Design review of the part built by this model. Coordinates are the model's own, in mm. A direction names the side the tool comes from. Give positions to 0.01 mm unless a question says otherwise; leave off trailing zeros. Loops run counter-clockwise (first coordinate to the right, second up) from the corner with the lowest first, then second, coordinate; pieces in that order, holes last. Notation, with made-up numbers: (-25.75, 79) - (1.25, 79) arc R14 ccw to (1.25, 84) - close; hole circle Ø11 at (64, 24). An arc over 180 degrees is marked (long way). Write each question's results on one line, items separated by ' | '.
from build123d import *

# Parameters (mm, degrees)
SKETCH_1_W          = 35.5
SKETCH_1_H          = 11
SKETCH_1_W_2        = 18.5
SKETCH_1_H_2        = 1.7
CUT_EXTRUDE_1_REACH = 79.86
SKETCH_2_R          = 1.5
CUT_EXTRUDE_START   = -4.5
CUT_EXTRUDE_3_DEPTH = 4.5
SKETCH_4_R          = 2
SKETCH_4_R_2        = 1.5
CUT_EXTRUDE_4_DEPTH = 5


with BuildPart() as part:
    # 草图1 → 旋转1 (revolve)
    with BuildSketch(Plane(origin=(0, 0, 0), x_dir=(1, 0, 0), z_dir=(0, 1, 0))):
        Polygon((0, 24.5), (0, 0), (35.5, 0), (49, 0), (49, 24.5), (24, 24.5), align=None)
        with Locations((17.75, -5.5)):
            Rectangle(SKETCH_1_W, SKETCH_1_H)
        Polygon((0, 25.8), (0, 24.5), (24, 24.5), (24, 25.8), (18.5, 25.8), align=None)
        with Locations((9.25, 26.65)):
            Rectangle(SKETCH_1_W_2, SKETCH_1_H_2)
    revolve(axis=Axis((0, 0, 11), (0, 0, -1)))

    # 草图2 → 切除-拉伸1 (cut, up to next)
    with BuildSketch(Plane(origin=(0, 0, -24.5), x_dir=(-1, 0, 0), z_dir=(0, 0, -1)), mode=Mode.PRIVATE) as cut_extrude_1_sk1:
        with Locations((16.264045876, 39.264880132)):
            Circle(SKETCH_2_R)
    cut_extrude_1_tool1 = extrude(cut_extrude_1_sk1.sketch, amount=-CUT_EXTRUDE_1_REACH, mode=Mode.PRIVATE) & part.part
    # 草图2 → 切除-拉伸1 (cut, up to next)
    with BuildSketch(Plane(origin=(0, 0, -24.5), x_dir=(-1, 0, 0), z_dir=(0, 0, -1)), mode=Mode.PRIVATE) as cut_extrude_1_sk2:
        with Locations((-16.264045876, 39.264880132)):
            Circle(SKETCH_2_R)
    cut_extrude_1_tool2 = extrude(cut_extrude_1_sk2.sketch, amount=-CUT_EXTRUDE_1_REACH, mode=Mode.PRIVATE) & part.part
    # 草图2 → 切除-拉伸1 (cut, up to next)
    with BuildSketch(Plane(origin=(0, 0, -24.5), x_dir=(-1, 0, 0), z_dir=(0, 0, -1)), mode=Mode.PRIVATE) as cut_extrude_1_sk3:
        with Locations((-39.264880132, 16.264045876)):
            Circle(SKETCH_2_R)
    cut_extrude_1_tool3 = extrude(cut_extrude_1_sk3.sketch, amount=-CUT_EXTRUDE_1_REACH, mode=Mode.PRIVATE) & part.part
    # 草图2 → 切除-拉伸1 (cut, up to next)
    with BuildSketch(Plane(origin=(0, 0, -24.5), x_dir=(-1, 0, 0), z_dir=(0, 0, -1)), mode=Mode.PRIVATE) as cut_extrude_1_sk4:
        with Locations((-39.264880132, -16.264045876)):
            Circle(SKETCH_2_R)
    cut_extrude_1_tool4 = extrude(cut_extrude_1_sk4.sketch, amount=-CUT_EXTRUDE_1_REACH, mode=Mode.PRIVATE) & part.part
    # 草图2 → 切除-拉伸1 (cut, up to next)
    with BuildSketch(Plane(origin=(0, 0, -24.5), x_dir=(-1, 0, 0), z_dir=(0, 0, -1)), mode=Mode.PRIVATE) as cut_extrude_1_sk5:
        with Locations((-16.264045876, -39.264880132)):
            Circle(SKETCH_2_R)
    cut_extrude_1_tool5 = extrude(cut_extrude_1_sk5.sketch, amount=-CUT_EXTRUDE_1_REACH, mode=Mode.PRIVATE) & part.part
    # 草图2 → 切除-拉伸1 (cut, up to next)
    with BuildSketch(Plane(origin=(0, 0, -24.5), x_dir=(-1, 0, 0), z_dir=(0, 0, -1)), mode=Mode.PRIVATE) as cut_extrude_1_sk6:
        with Locations((16.264045876, -39.264880132)):
            Circle(SKETCH_2_R)
    cut_extrude_1_tool6 = extrude(cut_extrude_1_sk6.sketch, amount=-CUT_EXTRUDE_1_REACH, mode=Mode.PRIVATE) & part.part
    # 草图2 → 切除-拉伸1 (cut, up to next)
    with BuildSketch(Plane(origin=(0, 0, -24.5), x_dir=(-1, 0, 0), z_dir=(0, 0, -1)), mode=Mode.PRIVATE) as cut_extrude_1_sk7:
        with Locations((39.264880132, -16.264045876)):
            Circle(SKETCH_2_R)
    cut_extrude_1_tool7 = extrude(cut_extrude_1_sk7.sketch, amount=-CUT_EXTRUDE_1_REACH, mode=Mode.PRIVATE) & part.part
    # 草图2 → 切除-拉伸1 (cut, up to next)
    with BuildSketch(Plane(origin=(0, 0, -24.5), x_dir=(-1, 0, 0), z_dir=(0, 0, -1)), mode=Mode.PRIVATE) as cut_extrude_1_sk8:
        with Locations((39.264880132, 16.264045876)):
            Circle(SKETCH_2_R)
    cut_extrude_1_tool8 = extrude(cut_extrude_1_sk8.sketch, amount=-CUT_EXTRUDE_1_REACH, mode=Mode.PRIVATE) & part.part
    add(cut_extrude_1_tool1.solids().sort_by_distance((-16.264046, 39.26488, -24.5))[0], mode=Mode.SUBTRACT)
    add(cut_extrude_1_tool2.solids().sort_by_distance((16.264046, 39.26488, -24.5))[0], mode=Mode.SUBTRACT)
    add(cut_extrude_1_tool3.solids().sort_by_distance((39.26488, 16.264046, -24.5))[0], mode=Mode.SUBTRACT)
    add(cut_extrude_1_tool4.solids().sort_by_distance((39.26488, -16.264046, -24.5))[0], mode=Mode.SUBTRACT)
    add(cut_extrude_1_tool5.solids().sort_by_distance((16.264046, -39.26488, -24.5))[0], mode=Mode.SUBTRACT)
    add(cut_extrude_1_tool6.solids().sort_by_distance((-16.264046, -39.26488, -24.5))[0], mode=Mode.SUBTRACT)
    add(cut_extrude_1_tool7.solids().sort_by_distance((-39.26488, -16.264046, -24.5))[0], mode=Mode.SUBTRACT)
    add(cut_extrude_1_tool8.solids().sort_by_distance((-39.26488, 16.264046, -24.5))[0], mode=Mode.SUBTRACT)

    # 草图3 → 切除-拉伸3 (cut)
    with BuildSketch(Plane.XY.offset(11).offset(CUT_EXTRUDE_START)):
        with BuildLine():
            Line((-38.5, 2.5), (-31.5, 2.5))
            ThreePointArc((-31.5, 2.5), (-29, 0), (-31.5, -2.5))
            Line((-31.5, -2.5), (-38.5, -2.5))
            ThreePointArc((-38.5, -2.5), (-41, 0), (-38.5, 2.5))
        make_face()
        with BuildLine():
            Line((-17.5, -30.886890423), (17.5, -30.886890423))
            ThreePointArc((17.5, -30.886890423), (0, -35.5), (-17.5, -30.886890423))
        make_face()
        with BuildLine():
            Line((-30.16456452, -24.962082865), (-25.214817051, -20.012335396))
            ThreePointArc((-25.214817051, -20.012335396), (-21.679283146, -20.012335396), (-21.679283146, -23.547869302))
            Line((-21.679283146, -23.547869302), (-26.629030614, -28.497616771))
            ThreePointArc((-26.629030614, -28.497616771), (-30.16456452, -28.497616771), (-30.16456452, -24.962082865))
        make_face()
        with BuildLine():
            Line((30.16456452, -24.962082865), (25.214817051, -20.012335396))
            ThreePointArc((25.214817051, -20.012335396), (21.679283146, -20.012335396), (21.679283146, -23.547869302))
            Line((21.679283146, -23.547869302), (26.629030614, -28.497616771))
            ThreePointArc((26.629030614, -28.497616771), (30.16456452, -28.497616771), (30.16456452, -24.962082865))
        make_face()
        with BuildLine():
            Line((38.5, 2.5), (31.5, 2.5))
            ThreePointArc((31.5, 2.5), (29, 0), (31.5, -2.5))
            Line((31.5, -2.5), (38.5, -2.5))
            ThreePointArc((38.5, -2.5), (41, 0), (38.5, 2.5))
        make_face()
        with BuildLine():
            Line((-30.16456452, 24.962082865), (-25.214817051, 20.012335396))
            ThreePointArc((-25.214817051, 20.012335396), (-21.679283146, 20.012335396), (-21.679283146, 23.547869302))
            Line((-21.679283146, 23.547869302), (-26.629030614, 28.497616771))
            ThreePointArc((-26.629030614, 28.497616771), (-30.16456452, 28.497616771), (-30.16456452, 24.962082865))
        make_face()
        with BuildLine():
            Line((30.16456452, 24.962082865), (25.214817051, 20.012335396))
            ThreePointArc((25.214817051, 20.012335396), (21.679283146, 20.012335396), (21.679283146, 23.547869302))
            Line((21.679283146, 23.547869302), (26.629030614, 28.497616771))
            ThreePointArc((26.629030614, 28.497616771), (30.16456452, 28.497616771), (30.16456452, 24.962082865))
        make_face()
    extrude(amount=CUT_EXTRUDE_3_DEPTH, mode=Mode.SUBTRACT)

    # 草图4 → 切除-拉伸4 (cut)
    with BuildSketch(Plane(origin=(0, 0, -27.5), x_dir=(-1, 0, 0), z_dir=(0, 0, -1))):
        with Locations((7, 12.124355653)):
            Circle(SKETCH_4_R)
        with Locations((14, 0)):
            Circle(SKETCH_4_R)
        with Locations((7, -12.124355653)):
            Circle(SKETCH_4_R)
        with Locations((-7, -12.124355653)):
            Circle(SKETCH_4_R)
        with Locations((-14, 0)):
            Circle(SKETCH_4_R)
        with Locations((-7, 12.124355653)):
            Circle(SKETCH_4_R)
        with Locations((0, 14)):
            Circle(SKETCH_4_R_2)
        with Locations((0, -14)):
            Circle(SKETCH_4_R_2)
    extrude(amount=-CUT_EXTRUDE_4_DEPTH, mode=Mode.SUBTRACT)


solid = part.part
(1) Take a section at A-A on x = 0. Give the boundary of the cut face in (y, z), plus the area to 3 significant figures.
Answers below:
outline: (-49, -24.5) - (-24, -24.5) - (-24, -25.8) - (-18.5, -25.8) - (-18.5, -27.5) - (-15.5, -27.5) - (-15.5, -22.5) - (-12.5, -22.5) - (-12.5, -27.5) - (12.5, -27.5) - (12.5, -22.5) - (15.5, -22.5) - (15.5, -27.5) - (18.5, -27.5) - (18.5, -25.8) - (24, -25.8) - (24, -24.5) - (49, -24.5) - (49, 0) - (35.5, 0) - (35.5, 11) - (-30.89, 11) - (-30.89, 6.5) - (-35.5, 6.5) - (-35.5, 0) - (-49, 0) - close | area: 3,260 mm2
(2) Take a section at B-B on z = 8.5. Give the boundary of the cut face in (x, y).
Answers below:
outline: (-35.41, -2.5) arc R35.5 ccw to (-27.57, -22.37) - (-25.21, -20.01) arc R2.5 cw to (-21.68, -23.55) - (-24.15, -26.02) arc R35.5 ccw to (-17.5, -30.89) - (17.5, -30.89) arc R35.5 ccw to (24.15, -26.02) - (21.68, -23.55) arc R2.5 cw to (25.21, -20.01) - (27.57, -22.37) arc R35.5 ccw to (35.41, -2.5) - (31.5, -2.5) arc R2.5 cw to (31.5, 2.5) - (35.41, 2.5) arc R35.5 ccw to (27.57, 22.37) - (25.21, 20.01) arc R2.5 cw to (21.68, 23.55) - (24.15, 26.02) arc R35.5 ccw to (-24.15, 26.02) - (-21.68, 23.55) arc R2.5 cw to (-25.21, 20.01) - (-27.57, 22.37) arc R35.5 ccw to (-35.41, 2.5) - (-31.5, 2.5) arc R2.5 cw to (-31.5, -2.5) - close
(3) Insertion check: P1, Ø5, axis at x = -12, z = -4.5, coming from the -Y side; P2, Ø2, axis at x = -21.5, z = -6.5, coming from the -Y side; P3, Ø5, axis at x = -39.26, y = 16.26, coming from the -Z side; P4, Ø2.5, axis at x = -0.5, y = 14.5, coming from the -Z side. Each pin has a flat end and moves straight along its axis. Give the tip position at first contact, or say it passes through.
Answers below:
P1: y = -48.07 | P2: y = -44.51 | P3: z = -24.5 | P4: z = -27.5
(4) Take a section at C-C on y = 4. Give the boundary of the cut face in (x, z), plus the area to 3 significant figures.
Answers below:
outline: (-48.84, -24.5) - (-23.66, -24.5) - (-23.66, -25.8) - (-18.06, -25.8) - (-18.06, -27.5) - (18.06, -27.5) - (18.06, -25.8) - (23.66, -25.8) - (23.66, -24.5) - (48.84, -24.5) - (48.84, 0) - (35.27, 0) - (35.27, 11) - (-35.27, 11) - (-35.27, 0) - (-48.84, 0) - close | area: 3,290 mm2
(5) Wall thickness on line 1 along Y through (x, z) = (0, -25); line 2 along Y through (x, z) = (0, -26.5); line 3 along Z through (x, y) = (-20, 21.5): over which ranges is each line inside the solid? List them lowest first. Write a range as from..to.
Answers below:
line 1: -24..-15.5, -12.5..12.5, 15.5..24 | line 2: -18.5..-15.5, -12.5..12.5, 15.5..18.5 | line 3: -24.5..11
(6) Tool access review of faces 1 (the flat face through (33, -2.5, 9)), 2 (the flat face through (-32, 0, 6.5)), 3 (the flat face through (-26.4, -21.2, 8.7)), 4 (the cylindrical face through (8.47, 13.48, -25.04)): name each direction out of +Z, -Z, +X, -X, +Y, -Y from which nothing blocks a thin tool from reaching the whole face with its end or side.
Answers below:
face 1: +Z, +X | face 2: +Z, -X | face 3: +Z, -Y | face 4: -Z
